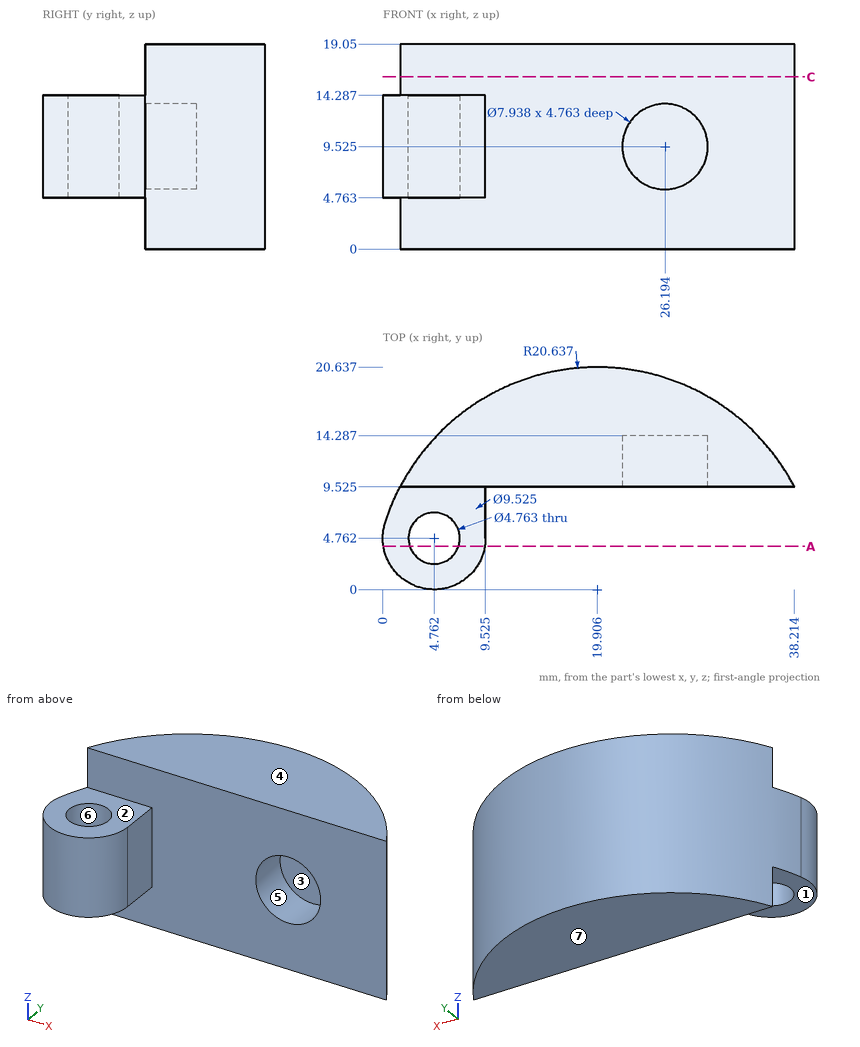
Input: dimensioned drawing with shaded views. Units: mm. Origin: part minimum x, y, z. A direction names the side the tool comes from. Round coordinates to 2 decimals unless told otherwise and drop trailing zeros. Loops run counter-clockwise (first coordinate to the right, second up) from the corner with the lowest first, then second, coordinate; pieces in that order, holes last. Notation, with made-up numbers: (58.25, 79) -> (87.25, 79) arc R19 ccw to (87.25, 83) -> close; hole circle Ø8 at (74, 64). An arc over 180 degrees is marked (long way). Answer as a JSON object with one key per item and string values. Group by question number.
Q1. Mould query, pull axis Z, two halves, no side actions, for the marked faces 4, 5, 6 and 7. Classes: pulls with the +Z half, pulls with the -Z half, needs draft (parallel to the pull), parting line crosses it, or undercut.
Q2. Ray query, line 1 (X direction, y = 3, z = 5.5) (1 decimal); line 2 (X direction, y = 3.5, z = 14) (1 decimal); line 3 (X direction, y = 14.25, z = 2.25) (1 decimal). Return the intervals inside material, ascending. Write a range as from..to.
Q3. Section query C-C (z = 16). Output: boundary loops of the cut face in (x, y) (1 decimal).
Q4. Contact query for flat-ended pins moving along their axis: P1, Ø3, axis at x = 5, y = 5, coming from the -Z side; P2, Ø5.5, axis at x = 4.76, y = 4.76, coming from the +Z side; P3, Ø3, axis at x = 26.5, z = 14.5, coming from the +Y side; P4, Ø1, axis at y = 9.5, z = 16, coming from the -X side. Output: stop coordinate, or through.
Q5. Access query for the marked faces 1, 2 and 3. Directions: +Z, -Z, +X, -X, +Y, -Y. A direction counts if a zero-diameter tool reaches every point of the face in a straight line with its end or side. Return the directions, or none.
Q6. Section query A-A (y = 4). Output: boundary loops of the cut face in (x, z).
Completed:
{
 "1": {"face 4": "pulls with the +Z half", "face 5": "undercut", "face 6": "needs draft", "face 7": "pulls with the -Z half"},
 "2": {"line 1": "0.3..3.2, 6.4..9.2", "line 2": "0.2..2.7, 6.8..9.4", "line 3": "5..34.8"},
 "3": {"outline": "(1.6, 9.5) -> (38.2, 9.5) arc R20.6 ccw to start"},
 "4": {"P1": "through", "P2": "z = 14.29", "P3": "y = 20", "P4": "x = 1.6"},
 "5": {"face 1": "-Z, +X, -X, -Y", "face 2": "+Z, +X, -X, -Y", "face 3": "-Y"},
 "6": {"outline": "(0.06, 4.76) -> (2.51, 4.76) -> (2.51, 14.29) -> (0.06, 14.29) -> close; (7.02, 4.76) -> (9.46, 4.76) -> (9.46, 14.29) -> (7.02, 14.29) -> close"}
}
